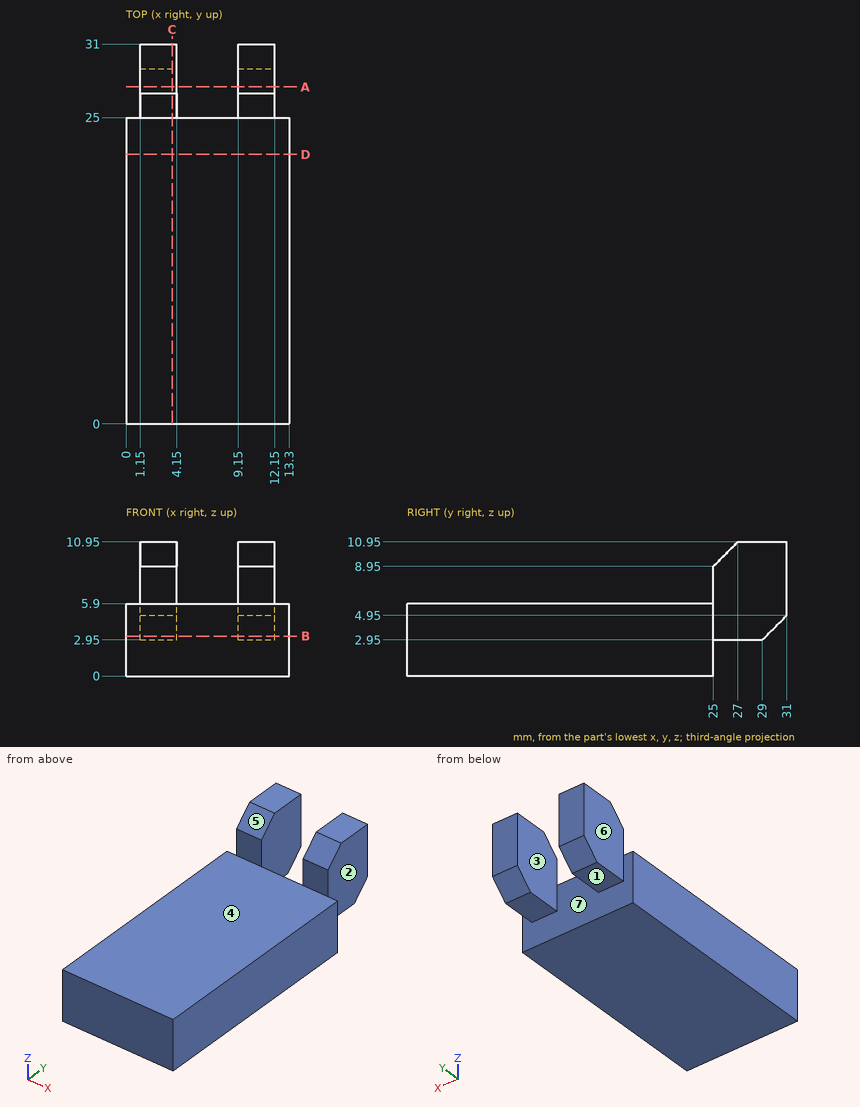
Source: three-view drawing plus pictorial views. Frame: mm from the lowest corner of the part. A direction names the side the tool comes from. Coordinates: 2 decimals unless noted, no trailing zeros. Order: outer loops, then holes, each group sorted by start corner. A loop starts at its lowest first (then second) coordinate and runs counter-clockwise, first axis right, second up. Notation, with made-up numbers: M 34,70 L 77,70 A17 cw 77,86 Z; hole C 27.5,57 d5. An arc over 180 degrees is marked long. Answer in a Markdown table with one row per item.
(1) Section query C-C, the plane x = 3.75. Output: boundary loops of the cut face in (y, z), plus the area to 4 significant figures.
Numbers:
| item | result |
|---|---|
| outline | M 0,0 L 25,0 L 25,2.95 L 29,2.95 L 31,4.95 L 31,10.95 L 27,10.95 L 25,8.95 L 25,5.9 L 0,5.9 Z |
| area | 191.5 mm^2 |
(2) Section query A-A, the plane y = 27.5. Output: boundary loops of the cut face in (x, z), plus the area to 3 significant figures.
Numbers:
| item | result |
|---|---|
| outline | M 1.15,2.95 L 4.15,2.95 L 4.15,10.95 L 1.15,10.95 Z; M 9.15,2.95 L 12.15,2.95 L 12.15,10.95 L 9.15,10.95 Z |
| area | 48.0 mm^2 |
(3) Draft query along X for the marked faces 5, 6 and 7. Return one class per face: pulls with the +X half, pulls with the -X half, needs draft (parallel to the pull), parting line crosses it, or undercut.
Numbers:
| item | result |
|---|---|
| face 5 | needs draft |
| face 6 | pulls with the -X half |
| face 7 | undercut |
(4) Section query B-B, the plane z = 3.25. Output: boundary loops of the cut face in (x, y).
Numbers:
| item | result |
|---|---|
| outline | M 0,0 L 13.3,0 L 13.3,25 L 12.15,25 L 12.15,29.3 L 9.15,29.3 L 9.15,25 L 4.15,25 L 4.15,29.3 L 1.15,29.3 L 1.15,25 L 0,25 Z |
(5) Section query D-D, the plane y = 22. Output: boundary loops of the cut face in (x, z).
Numbers:
| item | result |
|---|---|
| outline | M 0,0 L 13.3,0 L 13.3,5.9 L 0,5.9 Z |
(6) Contact query for flat-ended pins moving along their axis: pin 1 Ø5 at (x, y) = (5.5, 5) entering from -Z; pin 2 Ø3 at (y, z) = (26.5, 8) entering from +X; pin 3 Ø1.8 at (x, z) = (7, 2.5) entering from +Y; pin 4 Ø4 at (x, y) = (8, 14.5) entering from +Z. Output: stop coordinate, or through.
Numbers:
| item | result |
|---|---|
| pin 1 | stops at z = 0 |
| pin 2 | stops at x = 12.15 |
| pin 3 | stops at y = 25 |
| pin 4 | stops at z = 5.9 |
(7) Access query for the marked faces 1, 2, 3 and 4. Directions: +Z, -Z, +X, -X, +Y, -Y. A direction counts if a zero-diameter tool reaches every point of the face in a straight line with its end or side. Return the directions, or none.
Numbers:
| item | result |
|---|---|
| face 1 | -Z, +X, -X, +Y |
| face 2 | +Z, -Z, +X, +Y |
| face 3 | +Z, -Z, +Y |
| face 4 | +Z, +X, -X, -Y |
(8) Material intervals for line 1 (X direction, y = 29, z = 5); line 2 (Z direction, x = 8, y = 11); line 3 (Y direction, x = 9.5, z = 2), sorted ascending. Write a range as [from, to].
Numbers:
| item | result |
|---|---|
| line 1 | x = [1.15, 4.15], [9.15, 12.15] |
| line 2 | z = [0, 5.9] |
| line 3 | y = [0, 25] |
